Geometry check sheet. Reference: the model listing, model coordinates, mm. A direction names the side the tool comes from. Give positions to 0.01 mm unless a question says otherwise; leave off trailing zeros. Write each loop counter-clockwise with the first axis right and the second up, starting at its lowest first coordinate (ties: lowest second). Pieces come first, ordered by that corner, then holes. Notation, with made-up numbers: (41.5, 82) -> (92.5, 82) arc R31 ccw to (92.5, 106) -> close; hole circle Ø7 at (-27, 35.25). An arc over 180 degrees is marked (long way). One line per item, written item: value.
Autodesk Inventor part; units mm, degrees
ref_plane "YZ Plane" through (0, 0, 0) normal (1, 0, 0) x (0, 1, 0)
ref_plane "XZ Plane" through (0, 0, 0) normal (0, 1, 0) x (-1, 0, 0)
ref_plane "XY Plane" through (0, 0, 0) normal (0, 0, 1) x (1, 0, 0)
sketch "Boceto1" plane through (0, 0, 0) normal (0, 1, 0) x (-1, 0, 0)
  line L0 (80, 80) -> (0, 80)
  line L1 (0, 80) -> (0, 75)
  line L2 (80, 47.68) -> (80, 52.68)
  line L3 (80, 47.68) -> (80, 22.68)
  line L4 (80, 22.68) -> (75, 22.68)
  line L5 (75, 22.68) -> (71.4886, 22.68)
  line L6 (80, 80) -> (80, 52.68)
  arc A0 (71.4886, 22.68) -> (0, 75) centre (0, 0) ccw
  dimension "d4" = 5
  dimension "d5" = 25
extrude "Extrusión1" add sketch "Boceto1" along normal blind 20
sketch "Boceto2" plane through (-80, 0, 22.68) normal (-1, 0, 0) x (0, 0, 1)
  line L0 (0, 0) -> (52.32, 0)
  line L1 (25, 0) -> (30, 0)
  line L2 (30, 0) -> (30, 20)
  line L3 (0, 20) -> (52.32, 20)
  line L4 (25, 0) -> (25, 20)
  line L5 (25, 20) -> (30, 20)
  point P0 (-22.68, 0)
  dimension "d8" = 47.68
  dimension "d9" = 5
extrude "Extrusión2" add sketch "Boceto2" along normal blind 13
sketch "Boceto3" plane through (-80, 0, 47.68) normal (0, 0, -1) x (-1, 0, 0)
  line L0 (0, 0) -> (13, 0)
  line L1 (0, 0) -> (3, 0)
  line L2 (0, 20) -> (13, 20)
  line L3 (3, 15) -> (10, 15)
  line L4 (10, 15) -> (10, 5)
  line L5 (10, 5) -> (3, 5)
  line L6 (3, 5) -> (3, 15)
  point P0 (-80, 0)
  dimension "d12" = 3
  dimension "d14" = 7
  dimension "d15" = 10
extrude "Extrusión3" cut sketch "Boceto3" against normal blind 5
fillet "Empalme1" radius 30 1 edges at (-80, 10, 80)
fillet "Empalme2" radius 3 4 edges at (-80, 10, 22.68) (-71.4886, 10, 22.68) (0, 10, 75) (0, 10, 80)
properties part number "Positioner_Adapter"
1) Depth check by flat-ended pin: pin 1 Ø8 at (y, z) = (8, 38) entering from -X; pin 2 Ø2.5 at (y, z) = (7.5, 49.5) entering from +X; pin 3 Ø6 at (x, y) = (-81.5, 9) entering from -Z. Enter the tip coordinate at first touch or a pass-through.
Verdict:
pin 1: x = -80
pin 2: x = -55.22
pin 3: z = 23.08
2) Sectioned sample at B-B on x = -16. Record the cut outline in (y, z), plus the area to 3 significant figures.
Verdict:
outline: (0, 73.27) -> (20, 73.27) -> (20, 80) -> (0, 80) -> close
area: 135 mm^2
3) Mould release check, pull along Y, two halves, no side actions. Record for faces 1 (the flat face through (-57, 0, 62)), 2 (the cylindrical face through (-0.9, 9.9, 75.8)), 3 (the flat face through (-90, 10, 50)): released by +Y, released by -Y, zero draft, split by the parting line, or undercut.
Verdict:
face 1: released by -Y
face 2: zero draft
face 3: undercut
4) Sectioned sample at C-C on z = 46. Record the cut outline in (x, y).
Verdict:
outline: (-80, 0) -> (-59.24, 0) -> (-59.24, 20) -> (-80, 20) -> close
5) Tool access check on faces 4 (the flat face through (-87, 5, 50)), 5 (the flat face through (-80, 10, 37)), 6 (the flat face through (-91, 10, 52.68)). Record the directions out of +Z, -Z, +X, -X, +Y, -Y that give a thin tool (end or side, any length) a straight path to the whole face; none if there is none.
Verdict:
face 4: +Z, -Z
face 5: -Z, -X, +Y, -Y
face 6: +Z, -X, +Y, -Y
6) Scan lines: probe 1 along X at (y, z) = (6, 49); probe 2 along Z at (x, y) = (-28, 12.5); probe 3 along Z at (x, y) = (-32, 15). Record each from-to range of solid material in increasing order.
Verdict:
probe 1: -93 to -90, -83 to -56.78
probe 2: 69.58 to 80
probe 3: 67.83 to 80
7) Sectioned sample at A-A on y = 14. Record the cut outline in (x, z).
Verdict:
outline: (-93, 47.68) -> (-90, 47.68) -> (-90, 52.68) -> (-93, 52.68) -> close; (-83, 47.68) -> (-80, 47.68) -> (-80, 25.68) arc R3 ccw to (-77, 22.68) -> (-73.65, 22.68) arc R3 ccw to (-70.82, 24.69) arc R75 cw to (-2.88, 74.94) arc R3 ccw to (0, 77.94) arc R3 ccw to (-2.85, 80) -> (-50.12, 80) arc R30 ccw to (-80, 52.68) -> (-83, 52.68) -> close
